The listing builds one solid part. Answer for the finished solid, in the listing's coordinates (mm). A direction names the side the tool comes from. Give positions to 0.01 mm unless a question says otherwise; leave off trailing zeros. Write each loop counter-clockwise with the first axis right and the second up, starting at its lowest first coordinate (ties: lowest second). Pieces come first, ordered by that corner, then holes. Notation, with made-up numbers: (29.5, 35.5) - (56.5, 35.5) arc R20 cw to (56.5, 49.5) - close; hole circle Ø1 at (46.25, 15). An arc over 180 degrees is marked (long way). Answer as CSV lines item,"result". Start each with the question number.
(1) Each of these flat-tipped pins is pushed along its axis until it touches: pin 1 Ø1 at (x, y) = (3.5, 8.5) entering from -Z; pin 2 Ø8 at (y, z) = (2, 18.5) entering from -X; pin 3 Ø4 at (x, y) = (12.5, 10.5) entering from +Z; pin 4 Ø10 at (y, z) = (-13.5, 47) entering from -X. Where does it stop, or does it pass through?
(2) For a pull along Z with two mould halves and no side action, classify faces 1 (the face through (-2.17, -9.76, 56.48)), 2 (the face through (-0.867, -3.905, 28.636)), 3 (the face through (0, -4, 0)) as pulls with the +Z half, pulls with the -Z half, needs draft (parallel to the pull), parting line crosses it, or undercut.
(3) Find section A-A (x = 0). Write down the section's boundary in (y, z).
(4) Find section D-D (x = 8). Write down the section's boundary in (y, z).
(5) Straight lines are drawn through the part: probe 1 along Z at (x, y) = (1.5, -5); probe 2 along Y at (x, z) = (0, 24.5); probe 3 along Z at (x, y) = (15, -4.5). For each, find the intervals that lie inside material, in ascending order.
(6) For faces 4 (the face through (-0.1, -4.3, 55)), 5 (the face through (-13.887, -10.648, 1.479)), determine the directions among +Z, -Z, +X, -X, +Y, -Y from which every point of the face is accessible in a straight line to the end or side of a thin tool.
(7) Find section C-C (z = 41). Write down the section's boundary in (x, y).
from build123d import *

# Parameters (mm, degrees)
F0_R     = 17.5
F0_R_2   = 4
F1_DEPTH = 3
F2_DEPTH = 55
F3_R     = 10
F3_R_2   = 4
F4_DEPTH = 3
F5_R     = 1.5
F6_DEPTH = 58.001


with BuildPart() as f1:
    # F0 (on Top) → F1 (new body)
    with BuildSketch(Plane.XY):
        Circle(F0_R)
        Circle(F0_R_2, mode=Mode.SUBTRACT)
        Circle(F0_R_2)
    extrude(amount=F1_DEPTH)

    # F0 (on Top) → F2 (join)
    with BuildSketch(Plane.XY):
        Circle(F0_R_2)
    extrude(amount=F2_DEPTH)

    # F3 (on face) → F4 (join)
    with BuildSketch(Plane.XY.offset(55)):
        Circle(F3_R)
        Circle(F3_R_2)
    extrude(amount=F4_DEPTH)

    # F5 (on face) → F6 (cut, through all)
    with BuildSketch(Plane.XY.offset(58)):
        Circle(F5_R)
    extrude(amount=-F6_DEPTH, mode=Mode.SUBTRACT)


solid = f1.part
Result set:
1,pin 1,"z = 0"
1,pin 2,"x = -4"
1,pin 3,"z = 3"
1,pin 4,"through"
2,face 1,"needs draft"
2,face 2,"undercut"
2,face 3,"pulls with the -Z half"
3,outline,"(-17.5, 0) - (-1.5, 0) - (-1.5, 58) - (-10, 58) - (-10, 55) - (-4, 55) - (-4, 3) - (-17.5, 3) - close; (1.5, 0) - (17.5, 0) - (17.5, 3) - (4, 3) - (4, 55) - (10, 55) - (10, 58) - (1.5, 58) - close"
4,outline,"(-15.56, 0) - (15.56, 0) - (15.56, 3) - (-15.56, 3) - close; (-6, 55) - (6, 55) - (6, 58) - (-6, 58) - close"
5,probe 1,"0 to 3, 55 to 58"
5,probe 2,"-4 to -1.5, 1.5 to 4"
5,probe 3,"0 to 3"
6,face 4,"none"
6,face 5,"+Z, -Z"
7,outline,"circle Ø8 at (0, 0); hole circle Ø3 at (0, 0)"
